Input: dimensioned drawing with shaded views. Units: mm. Origin: part minimum x, y, z. Round coordinates to 2 decimals unless told otherwise and drop trailing zeros. Write each loop counter-clockwise with the first axis right and the second up, starting at its lowest first coordinate (ties: lowest second). Pieces come first, ordered by that corner, then holes. Notation, with made-up numbers: (72, 65.25) - (93, 65.25) arc R26 cw to (93, 81.25) - close; hole circle Ø10 at (-2.5, 23). An arc over 180 degrees is marked (long way). Use one line per item in the form item = value.
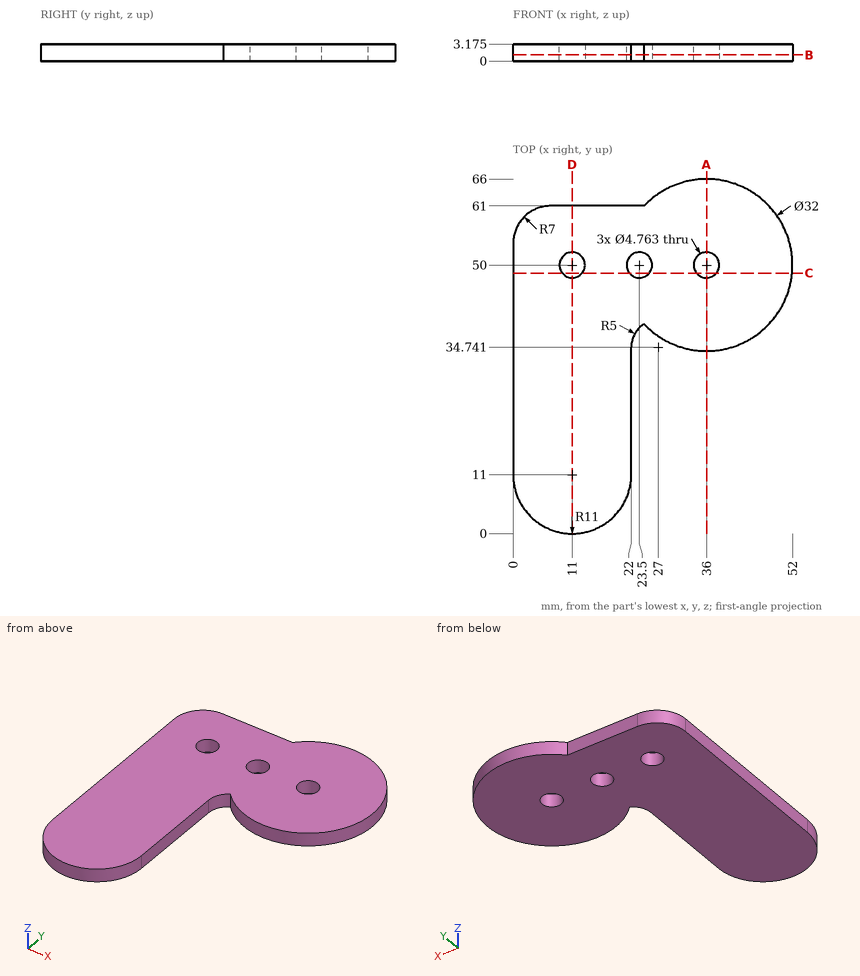
(1) Material intervals for L1, parallel to Y at x = 11, z = 2.2; L2, parallel to X at y = 25, z = 1.45; L3, parallel to X at y = 49.5, z = 2.25, sorted ascending.
Derived:
L1 = 0 to 47.62, 52.38 to 61
L2 = 0 to 22
L3 = 0 to 8.67, 13.33 to 21.17, 25.83 to 33.67, 38.33 to 51.99
(2) Cut plane D-D on x = 11. Output: boundary loops of the cut face in (y, z) (1 decimal).
Derived:
outline = (0, 0) - (47.6, 0) - (47.6, 3.2) - (0, 3.2) - close; (52.4, 0) - (61, 0) - (61, 3.2) - (52.4, 3.2) - close
(3) Cut plane C-C on y = 48.5. Count the separate pieces of the cut face and the enclosed holes in it, then the cut area to 3 significant figures.
Derived:
separate_pieces = 4
enclosed_holes = 0
area = 130 mm^2
(4) First-contact query: pin 1 Ø1.6 at (x, z) = (20, 2) entering from +Y; pin 2 Ø1 at (y, z) = (51.5, 0.5) entering from +X; pin 3 Ø4 at (x, y) = (11, 50) entering from -Z; pin 4 Ø1.6 at (y, z) = (19.5, 2) entering from +X. Flat tips, straight axial feed; report the tip coordinate or a pass-through.
Derived:
pin_1 = 61
pin_2 = 51.97
pin_3 = through
pin_4 = 22
(5) Cut plane B-B on z = 1.15. Output: boundary loops of the cut face in (x, y), then the cut area to 3 significant figures.
Derived:
outline = (0, 11) arc R11 ccw to (22, 11) - (22, 34.74) arc R5 cw to (24.38, 39) arc R16 ccw (long way) to (24.38, 61) - (7, 61) arc R7 ccw to (0, 54) - close; hole circle Ø4.76 at (11, 50); hole circle Ø4.76 at (23.5, 50); hole circle Ø4.76 at (36, 50)
area = 2,020 mm^2
(6) Cut plane A-A on x = 36. Output: boundary loops of the cut face in (y, z) (1 decimal).
Derived:
outline = (34, 0) - (47.6, 0) - (47.6, 3.2) - (34, 3.2) - close; (52.4, 0) - (66, 0) - (66, 3.2) - (52.4, 3.2) - close
